Autodesk Inventor part; units mm, degrees
ref_plane "YZ Plane" through (0, 0, 0) normal (1, 0, 0) x (0, 1, 0)
ref_plane "XZ Plane" through (0, 0, 0) normal (0, 1, 0) x (-1, 0, 0)
ref_plane "XY Plane" through (0, 0, 0) normal (0, 0, 1) x (1, 0, 0)
sketch "Sketch1" plane through (0, 0, 0) normal (0, 0, 1) x (1, 0, 0)
  line L0 (-3.6662, 6.35) -> (3.6662, 6.35)
  line L1 (3.6662, 6.35) -> (7.3323, 0)
  line L2 (7.3323, 0) -> (3.6662, -6.35)
  line L3 (3.6662, -6.35) -> (-3.6662, -6.35)
  line L4 (-3.6662, -6.35) -> (-7.3323, 0)
  line L5 (-7.3323, 0) -> (-3.6662, 6.35)
  point P0 (0, 0)
  point P1 (0, 0)
  dimension "d0" = 12.7
extrude "Extrusion1" add sketch "Sketch1" along normal mid plane 25.4
sketch "Sketch2" plane through (0, 0, 12.7) normal (0, 0, 1) x (1, 0, 0)
  point P0 (0, 0)
  point P1 (0, 0)
hole "Hole1" at (0, 0, 12.7) direction (0, 0, -1) diameter 4.9784 end through all
properties part number "Hex Standoff 14-20 x1000" material "Aluminum 6061"
Can you work these out from the model? Positions are in its coordinate system, mm. Round coordinates to 2 decimals unless told otherwise and drop trailing zeros. Loops run counter-clockwise (first coordinate to the right, second up) from the corner with the lowest first, then second, coordinate; pieces in that order, holes last. Notation, with made-up numbers: (28.25, 2) - (80.25, 2) arc R15 cw to (80.25, 27) - close; hole circle Ø7 at (-37.75, 29.25). An arc over 180 degrees is marked (long way). Use CSV: the item, a comma, the result in double quotes. Start each with the question number.
1) Please list where these lines run through material, in increasing order: probe 1 along Y at (x, z) = (0, 7.5); probe 2 along Y at (x, z) = (1, 0.25); probe 3 along X at (y, z) = (-1.25, 9). Write a range as [from, to].
2) We'd pull the mould along X, two halves only. Please class faces 1 (the flat face through (5.474, 3.219, -0.178)), 2 (the flat face through (3, 0, -12.7)), 3 (the cylindrical face through (-0.748, -2.374, -0.178)): released by +X, released by -X, zero draft, split by the parting line, or undercut.
3) If we section it at D-D on x = 5.25: Write out the boundary of the cut face in (y, z), plus the area to 3 significant figures.
4) If we section it at C-C on z = 10: Write out the boundary of the cut face in (x, y).
5) If we section it at B-B on y = 1: Write out the boundary of the cut face in (x, z).
6) If we section it at A-A on x = 0: Write out the boundary of the cut face in (y, z).
Geometry results:
1,probe 1,"y = [-6.35, -2.49], [2.49, 6.35]"
1,probe 2,"y = [-6.35, -2.28], [2.28, 6.35]"
1,probe 3,"x = [-6.61, -2.15], [2.15, 6.61]"
2,face 1,"released by +X"
2,face 2,"zero draft"
2,face 3,"undercut"
3,outline,"(-3.61, -12.7) - (3.61, -12.7) - (3.61, 12.7) - (-3.61, 12.7) - close"
3,area,"183 mm2"
4,outline,"(-7.33, 0) - (-3.67, -6.35) - (3.67, -6.35) - (7.33, 0) - (3.67, 6.35) - (-3.67, 6.35) - close; hole circle Ø4.98 at (0, 0)"
5,outline,"(-6.75, -12.7) - (-2.28, -12.7) - (-2.28, 12.7) - (-6.75, 12.7) - close; (2.28, -12.7) - (6.75, -12.7) - (6.75, 12.7) - (2.28, 12.7) - close"
6,outline,"(-6.35, -12.7) - (-2.49, -12.7) - (-2.49, 12.7) - (-6.35, 12.7) - close; (2.49, -12.7) - (6.35, -12.7) - (6.35, 12.7) - (2.49, 12.7) - close"
